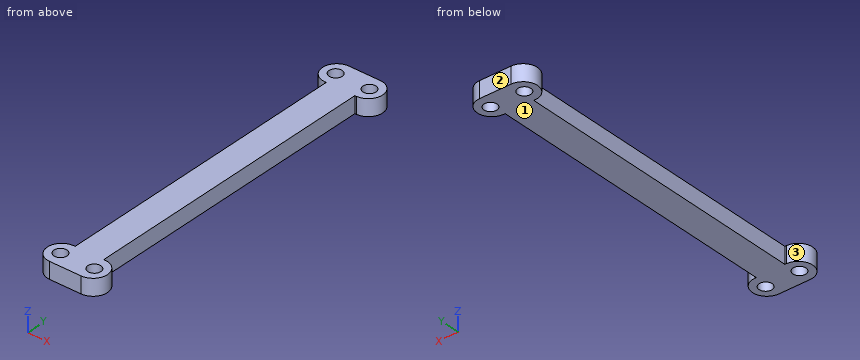
```python
from build123d import *

# Parameters (mm, degrees)
SKETCH_R  = 1.58
PAD_DEPTH = 4


with BuildPart() as part:
    # Sketch → Pad (new body)
    with BuildSketch(Plane.XY):
        with BuildLine():
            Line((-3.48, 0), (-3.48, 36.3))
            Line((-3.48, 36.3), (-3.81555, 36.3))
            ThreePointArc((-3.81555, 43.26), (-7.29555, 39.78), (-3.81555, 36.3))
            Line((-3.81555, 43.26), (3.81555, 43.26))
            ThreePointArc((3.81555, 36.3), (7.29555, 39.78), (3.81555, 43.26))
            Line((3.48, 36.3), (3.81555, 36.3))
            Line((3.48, 0), (3.48, 36.3))
            Line((-3.48, 0), (3.48, 0))
        make_face()
        with Locations((-4.11555, 39.78)):
            Circle(SKETCH_R, mode=Mode.SUBTRACT)
        with Locations((4.11555, 39.78)):
            Circle(SKETCH_R, mode=Mode.SUBTRACT)
    pad = extrude(amount=PAD_DEPTH)

    # Mirrored: Pad across Sketch H_Axis
    add(pad.mirror(Plane.ZX))


solid = part.part
```
Can you work these out from the model? Positions are in its coordinate system, mm. Face numbers are marked on the shaded views. Give positions to 0.01 mm unless a question says otherwise; leave off trailing zeros. Order: outer loops, then holes, each group sorted by start corner. A loop starts at its lowest first (then second) coordinate and runs counter-clockwise, first axis right, second up. Notation, with made-up numbers: M 72,44.25 L 108,44.25 A30 cw 108,69.25 Z; hole C 17,27.5 d8. An arc over 180 degrees is marked long. Write item = value, one per line. Start each with the question number.
Q1. Will these pins go through, and if not, where does the flat tip stop? pin 1 Ø2.5 at (x, y) = (4.12, -39.78) entering from -Z; pin 2 Ø2 at (x, z) = (-5.5, 3) entering from +Y; pin 3 Ø2 at (y, z) = (12.5, 2.5) entering from +X; pin 4 Ø1.5 at (y, z) = (19.5, 2.5) entering from -X.
Q2. Suppose I cut it at C-C (x = -4.75). Write out the boundary of the cut face in (y, z).
Q3. I need wall thicknesses on probe 1 along Y at (x, z) = (4, 1.7); probe 2 along X at (y, z) = (-39.78, 2.4); probe 3 along Y at (x, z) = (5.5, 0.35). Which ranges of each line are inside material? Lowest first, please. Write a range as [from, to].
Q4. We'd pull the mould along Y, two halves only. Please class the marked faces 1, 2 and 3: pulls with the +Y half, pulls with the -Y half, needs draft (parallel to the pull), parting line crosses it, or undercut.
Q5. Suppose I cut it at D-D (y = 11.5). Write out the boundary of the cut face in (x, z), plus the area to 3 significant figures.
Q6. Suppose I cut it at A-A (y = -39.78). Write out the boundary of the cut face in (x, z), plus the area to 3 significant figures.
Q7. Suppose I cut it at B-B (z = 1.1). Write out the boundary of the cut face in (x, y).
Check result:
q1.pin_1 = through
q1.pin_2 = 43.19
q1.pin_3 = 3.48
q1.pin_4 = -3.48
q2.outline = M -43.13,0 L -41.23,0 L -41.23,4 L -43.13,4 Z; M -38.33,0 L -36.43,0 L -36.43,4 L -38.33,4 Z; M 36.43,0 L 38.33,0 L 38.33,4 L 36.43,4 Z; M 41.23,0 L 43.13,0 L 43.13,4 L 41.23,4 Z
q3.probe_1 = [-43.26, -41.36], [-38.2, -36.3], [36.3, 38.2], [41.36, 43.26]
q3.probe_2 = [-7.3, -5.7], [-2.54, 2.54], [5.7, 7.3]
q3.probe_3 = [-42.83, -40.54], [-39.02, -36.73], [36.73, 39.02], [40.54, 42.83]
q4.face_1 = needs draft
q4.face_2 = pulls with the +Y half
q4.face_3 = undercut
q5.outline = M -3.48,0 L 3.48,0 L 3.48,4 L -3.48,4 Z
q5.area = 27.8 mm2
q6.outline = M -7.3,0 L -5.7,0 L -5.7,4 L -7.3,4 Z; M -2.54,0 L 2.54,0 L 2.54,4 L -2.54,4 Z; M 5.7,0 L 7.3,0 L 7.3,4 L 5.7,4 Z
q6.area = 33.1 mm2
q7.outline = M -3.82,-43.26 L 3.82,-43.26 A3.48 ccw 3.82,-36.3 L 3.48,-36.3 L 3.48,36.3 L 3.82,36.3 A3.48 ccw 3.82,43.26 L -3.82,43.26 A3.48 ccw -3.82,36.3 L -3.48,36.3 L -3.48,-36.3 L -3.82,-36.3 A3.48 ccw Z; hole C -4.12,-39.78 d3.16; hole C -4.12,39.78 d3.16; hole C 4.12,-39.78 d3.16; hole C 4.12,39.78 d3.16
